Model file for the job. Use its own axes, mm. A direction names the side the tool comes from. Coordinates: 2 decimals unless noted, no trailing zeros. Write each loop counter-clockwise with the first axis right and the second up, starting at its lowest first coordinate (ties: lowest second). Pieces come first, ordered by that corner, then holes. Notation, with made-up numbers: M 84.25,35 L 128.25,35 A33 ccw 128.25,74 Z; hole C 70.5,-36.75 d7. An arc over 180 degrees is marked long. Put each result on its own line as item: value. Start each with the question number.
Q1. Cut at B-B (y = 4.75). Write the cut outline in (x, z).
Q2. Drill centre lines: line 1 along X through (y, z) = (5, -28.5); line 2 along Z through (x, y) = (-17.5, 3.75); line 3 along Y through (x, z) = (-9.5, -18.5). Where is each one in solid material? Low to high.
Q3. Drop flat-ended pins along their axis: pin 1 (1.3 mm diameter, centred on x = -3.5, y = 5, fed in from +Z); pin 2 (3 mm diameter, centred on x = -16.06, z = -31.06, fed in from -Y); pin 3 (4.5 mm diameter, centred on x = -16.06, z = -31.06, fed in from +Y). Give the stop position or say it passes through.
Q4. Pull direction Z, two halves, no side cores. Call faces 4 (the flat face through (-22.5, 5, 0)), 5 (the flat face through (0, 5, -34.026)), 6 (the cylindrical face through (23.95, 3.25, -36.5)): pulls with the +Z half, pulls with the -Z half, needs draft (parallel to the pull), parting line crosses it, or undercut.
Q5. Which spindle directions (+Z, -Z, +X, -X, +Y, -Y) get a long thin tool onto all of the face, cutting with end or side? Do faces 1 (the flat face through (0, 5, -35.026)), 2 (the cylindrical face through (-18.238, 3.254, -29.382)), 3 (the cylindrical face through (24.14, 0.9, -0.48)). Say none if no direction does.
Q6. Cut at D-D (y = 1.5). Give the number of separate pieces and of enclosed holes in the cut face, then the cut area to 3 significant figures.
Autodesk Inventor part; units mm, degrees
ref_plane "YZ Plane" through (0, 0, 0) normal (1, 0, 0) x (0, 1, 0)
ref_plane "XZ Plane" through (0, 0, 0) normal (0, 1, 0) x (-1, 0, 0)
ref_plane "XY Plane" through (0, 0, 0) normal (0, 0, 1) x (1, 0, 0)
sketch "Sketch1" plane through (0, 0, 0) normal (0, 1, 0) x (-1, 0, 0)
  line L0 (-25, 37.5) -> (25, 37.5)
  line L1 (25, 37.5) -> (25, -37.5)
  line L2 (25, -37.5) -> (-25, -37.5)
  line L3 (-25, -37.5) -> (-25, 37.5)
  line L4 (25, 37.5) -> (-25, -37.5) construction
  line L5 (-22.5, 35) -> (22.5, 35)
  line L6 (22.5, 35) -> (22.5, -35)
  line L7 (22.5, -35) -> (-22.5, -35)
  line L8 (-22.5, -35) -> (-22.5, 35)
  line L9 (22.5, 35) -> (-22.5, -35) construction
  line L10 (22.5, 35) -> (20, 35)
  line L11 (20, 35) -> (20, 32.5)
  line L12 (20, 32.5) -> (22.5, 32.5)
  line L13 (22.5, 32.5) -> (22.5, 35)
  arc A0 (22.5, 32.5) -> (20, 35) centre (20, 32.5) ccw
  line L14 (25, 37.5) -> (21.5, 37.5)
  line L15 (21.5, 37.5) -> (21.5, 34)
  line L16 (21.5, 34) -> (25, 34)
  line L17 (25, 34) -> (25, 37.5)
  line L18 (22.5, -35) -> (20, -35)
  line L19 (20, -35) -> (20, -32.5)
  line L20 (20, -32.5) -> (22.5, -32.5)
  line L21 (22.5, -32.5) -> (22.5, -35)
  line L22 (-22.5, -35) -> (-20, -35)
  line L23 (-20, -35) -> (-20, -32.5)
  line L24 (-20, -32.5) -> (-22.5, -32.5)
  line L25 (-22.5, -32.5) -> (-22.5, -35)
  line L26 (-22.5, 35) -> (-20, 35)
  line L27 (-20, 35) -> (-20, 32.5)
  line L28 (-20, 32.5) -> (-22.5, 32.5)
  line L29 (-22.5, 32.5) -> (-22.5, 35)
  arc A1 (-20, 35) -> (-22.5, 32.5) centre (-20, 32.5) ccw
  arc A2 (-22.5, -32.5) -> (-20, -35) centre (-20, -32.5) ccw
  arc A3 (20, -35) -> (22.5, -32.5) centre (20, -32.5) ccw
  arc A4 (25, 34) -> (21.5, 37.5) centre (21.5, 34) ccw
  line L30 (25, -37.5) -> (21.5, -37.5)
  line L31 (21.5, -37.5) -> (21.5, -34)
  line L32 (21.5, -34) -> (25, -34)
  line L33 (25, -34) -> (25, -37.5)
  line L34 (-25, -37.5) -> (-21.5, -37.5)
  line L35 (-21.5, -37.5) -> (-21.5, -34)
  line L36 (-21.5, -34) -> (-25, -34)
  line L37 (-25, -34) -> (-25, -37.5)
  line L38 (-25, 37.5) -> (-21.5, 37.5)
  line L39 (-21.5, 37.5) -> (-21.5, 34)
  line L40 (-21.5, 34) -> (-25, 34)
  line L41 (-25, 34) -> (-25, 37.5)
  arc A5 (-21.5, 37.5) -> (-25, 34) centre (-21.5, 34) ccw
  arc A6 (-25, -34) -> (-21.5, -37.5) centre (-21.5, -34) ccw
  arc A7 (21.5, -37.5) -> (25, -34) centre (21.5, -34) ccw
  point P0 (0, 0)
  point P1 (25, 34)
  point P2 (-25, -34)
  point P3 (-22.5, -32.5)
  point P4 (-22, -34)
  point P5 (-22.5, -34)
  point P6 (22.5, -32.5)
  dimension "d0" = 50
  dimension "d1" = 75
  dimension "d2" = 45
  dimension "d3" = 70
  dimension "d8" = 2.5
  dimension "d9" = 2.5
extrude "Extrusion3" add sketch "Sketch1" along normal blind 3.5 contours L0 L15 L5 L39 | L39 L5 L8 L40 A5 | L40 L8 L36 L3 | A4 L16 L6 L5 L15 | L39 A1 L40 L8 L5 | L5 A1 L39 | L36 L8 L7 L35 A6 | L40 A1 L8 | L15 A0 L5 | L5 L6 L16 A0 L15 | L1 L32 L6 L16 | L5 L11 L12 L6 L20 L19 L7 L23 L24 L8 L28 L27 | L27 L28 A1 L40 L39 | L39 L40 A1 | L36 A2 L35 L7 L8 | L8 A2 L36 | L35 L7 L31 L2 | A0 L15 L16 L12 L11 | A0 L16 L15 | A7 L31 L7 L6 L32 | L6 A0 L16 | L24 L23 A2 L35 L36 | L36 L35 A2 | L35 A2 L7 | L32 A3 L6 | L6 L7 L31 A3 L32 | L7 A3 L31 | A3 L32 L31 L19 L20 | A3 L31 L32
fillet "Fillet1" radius 3 8 edges at (-23.9749, 0, 36.4749) (0, 0, 37.5) (23.9749, 0, 36.4749) (25, 0, 0) (23.9749, 0, -36.4749) (0, 0, -37.5) (-23.9749, 0, -36.4749) (-25, 0, 0)
sketch "Sketch2" plane through (0, 3.5, 0) normal (0, 1, 0) x (1, 0, 0)
  arc A0 (20, 32.5) -> (17.5, 35) centre (17.5, 32.5) ccw
  line L0 (17.5, 35) -> (17.5, 33.5)
  line L1 (20, -32.5) -> (20, 32.5)
  line L2 (20, 32.5) -> (18.5, 32.5)
  line L3 (18.5, 32.5) -> (17.5, 33.5)
  line L4 (18, 33) -> (16.0555, 31.0555)
  circle A1 centre (16.0555, 31.0555) radius 2.75
  line L5 (-20, 32.5) -> (-20, -32.5)
  line L6 (-20, -32.5) -> (-18.5, -32.5)
  line L7 (-17.5, -35) -> (17.5, -35)
  line L8 (-17.5, -35) -> (-17.5, -33.5)
  line L9 (-17.5, -33.5) -> (-18.5, -32.5)
  line L10 (-18, -33) -> (-16.0555, -31.0555)
  line L11 (-18, -33) -> (-15.25, -33) construction
  circle A2 centre (-16.0555, -31.0555) radius 2.75
  arc A3 (17.5812, 28.7675) -> (18.8055, 31.0555) centre (16.0555, 31.0555) ccw construction
  arc A4 (17.8504, 28.3639) -> (19.2906, 31.0555) centre (16.0555, 31.0555) ccw
  arc A5 (17.3121, 29.1712) -> (18.3203, 31.0555) centre (16.0555, 31.0555) ccw
  arc A6 (17.3121, 29.1712) -> (17.8504, 28.3639) centre (17.5812, 28.7675) ccw
  arc A7 (19.2906, 31.0555) -> (18.3203, 31.0555) centre (18.8055, 31.0555) ccw
  arc A8 (14.2605, 33.747) -> (12.8203, 31.0555) centre (16.0555, 31.0555) ccw
  arc A9 (12.8203, 31.0555) -> (13.7906, 31.0555) centre (13.3055, 31.0555) ccw
  arc A10 (14.7989, 32.9398) -> (14.2605, 33.747) centre (14.5297, 33.3434) ccw
  arc A11 (14.7989, 32.9398) -> (13.7906, 31.0555) centre (16.0555, 31.0555) ccw
  arc A12 (-14.2605, -33.747) -> (-12.8203, -31.0555) centre (-16.0555, -31.0555) ccw
  arc A13 (-14.7989, -32.9398) -> (-13.7906, -31.0555) centre (-16.0555, -31.0555) ccw
  arc A14 (-14.7989, -32.9398) -> (-14.2605, -33.747) centre (-14.5297, -33.3434) ccw
  arc A15 (-12.8203, -31.0555) -> (-13.7906, -31.0555) centre (-13.3055, -31.0555) ccw
  arc A16 (-17.8504, -28.3639) -> (-19.2906, -31.0555) centre (-16.0555, -31.0555) ccw
  arc A17 (-19.2906, -31.0555) -> (-18.3203, -31.0555) centre (-18.8055, -31.0555) ccw
  arc A18 (-17.3121, -29.1712) -> (-17.8504, -28.3639) centre (-17.5812, -28.7675) ccw
  arc A19 (-17.3121, -29.1712) -> (-18.3203, -31.0555) centre (-16.0555, -31.0555) ccw
  line L12 (-19.2843, -34.2843) -> (-16.7157, -31.7157) construction
  line L13 (-18.86, -34.7085) -> (-16.2915, -32.14)
  line L14 (-17.14, -31.2915) -> (-19.7085, -33.86)
  arc A20 (-19.7085, -33.86) -> (-18.86, -34.7085) centre (-19.2843, -34.2843) ccw
  arc A21 (-16.2915, -32.14) -> (-17.14, -31.2915) centre (-16.7157, -31.7157) ccw
  line L15 (16.5205, 31.5205) -> (19.4795, 34.4795) construction
  line L16 (16.9448, 31.0962) -> (19.9038, 34.0552)
  line L17 (19.0552, 34.9038) -> (16.0962, 31.9448)
  arc A22 (16.0962, 31.9448) -> (16.9448, 31.0962) centre (16.5205, 31.5205) ccw
  arc A23 (19.9038, 34.0552) -> (19.0552, 34.9038) centre (19.4795, 34.4795) ccw
  circle A24 centre (16.0555, 31.0555) radius 1.25
  circle A25 centre (-16.0555, -31.0555) radius 1.25
  line L18 (21.5, 34.5) -> (-21.5, 34.5)
  line L19 (0, 34.5) -> (0, -35)
  circle A26 centre (16.0555, -31.0555) radius 2.75
  circle A27 centre (16.0555, -31.0555) radius 1.25
  circle A28 centre (-16.0555, 31.0555) radius 2.75
  circle A29 centre (-16.0555, 31.0555) radius 1.25
  point P0 (0, 0)
  point P1 (18.3774, 32.5289)
  point P2 (17.5289, 33.3774)
  point P3 (14.9555, 33.5759)
  point P4 (13.3482, 30.5722)
  point P5 (17.1554, 28.535)
  point P6 (18.7627, 31.5387)
  point P7 (-18.3774, -32.5289)
  point P8 (-17.5289, -33.3774)
  point P9 (-14.9555, -33.5759)
  point P10 (-13.3482, -30.5722)
  point P11 (-17.1554, -28.535)
  point P12 (-18.7627, -31.5387)
  dimension "d32" = 5.5
  dimension "d29" = 1.5
  dimension "d30" = 1.5
  dimension "d31" = 2.75
  dimension "d33" = 1.5
  dimension "d34" = 1.5
  dimension "d35" = 2.75
  dimension "d36" = 45
  dimension "d37" = 5.5
  dimension "d40" = 360
  dimension "d44" = 1.2
  dimension "d45" = 1.2
  dimension "d60" = 2.5
  dimension "d61" = 2.5
sketch "Sketch4" plane through (0, 3.5, 0) normal (0, 1, 0) x (1, 0, 0)
  line L0 (-22, 34.5263) -> (22, 34.5263)
  line L1 (22, 34.5263) -> (22, -34.5263)
  line L2 (22, -34.5263) -> (-22, -34.5263)
  line L3 (-22, -34.5263) -> (-22, 34.5263)
  line L4 (-22, 34.5263) -> (22, -34.5263) construction
  line L5 (22, 34.5263) -> (-22, -34.5263) construction
  line L6 (21.5, 34.5) -> (-21.5, 34.5)
  line L7 (-21.5, 34.5) -> (-21.5, 37.5)
  line L8 (17.5001, 34.5) -> (-21.5, 34.5) construction
  line L9 (22, -34) -> (22, 34)
  line L10 (22, 32.5003) -> (22, -34.5263) construction
  arc A0 (21.5, -34.5263) -> (22.5, -34.5263) centre (22, -34.5263) ccw
  line L11 (22, -34.5263) -> (-22, -34.5263) construction
  line L12 (22, -34.0263) -> (-22, -34.0263)
  line L13 (-22, -35.0263) -> (22, -35.0263)
  arc A1 (22, -35.0263) -> (22, -34.0263) centre (22, -34.5263) ccw
  arc A2 (-22, -34.0263) -> (-22, -35.0263) centre (-22, -34.5263) ccw
  line L14 (-22, -34.5263) -> (-22, 34.5263) construction
  line L15 (-21.5, -34.5263) -> (-21.5, 34.5263)
  line L16 (-22.5, 34.5263) -> (-22.5, -34.5263)
  arc A3 (-22.5, -34.5263) -> (-21.5, -34.5263) centre (-22, -34.5263) ccw
  arc A4 (-21.5, 34.5263) -> (-22.5, 34.5263) centre (-22, 34.5263) ccw
  line L17 (22, 34.5263) -> (-22, 34.5263) construction
  line L18 (22, 35.0263) -> (-22, 35.0263)
  line L19 (-22, 34.0263) -> (22, 34.0263)
  arc A5 (22, 34.0263) -> (22, 35.0263) centre (22, 34.5263) ccw
  arc A6 (-22, 35.0263) -> (-22, 34.0263) centre (-22, 34.5263) ccw
  line L20 (22, -34.5263) -> (22, 34.5263) construction
  line L21 (22.5, -34.5263) -> (22.5, 34.5263)
  line L22 (21.5, 34.5263) -> (21.5, -34.5263)
  arc A7 (21.5, -34.5263) -> (22.5, -34.5263) centre (22, -34.5263) ccw
  arc A8 (22.5, 34.5263) -> (21.5, 34.5263) centre (22, 34.5263) ccw
  point P0 (0, 0)
  point P1 (-1.9999, 34.5)
  point P2 (22, -1.013)
  point P3 (0, -34.5263)
  point P4 (-22, 0)
  point P5 (0, 34.5263)
  point P6 (22, 0)
  point P7 (-22.5, -34.5263)
  point P8 (22, -35.0263)
  point P9 (22.5, -34.5263)
  point P10 (22.5, 34.5263)
  point P11 (-21.5, -34.0263)
  point P12 (-21.5, 34.0263)
  point P13 (21.5, 34.0263)
  point P14 (21.5, -34.0263)
  dimension "d68" = 1
  dimension "d69" = 1
  dimension "d70" = 1
  dimension "d71" = 1
  dimension "d72" = 1
extrude "Extrusion11" add sketch "Sketch4" along normal blind 3 contours L3 A6 A4 L0 | L0 L7 L15 L19 L3 | L7 L18 A8 L0 | L0 L22 L6 L7 | A4 L18 L7 | L19 L15 L12 L3 | L3 A2 L16 A6 | A8 A5 L1 L0 | L0 L1 L19 L22 | L6 L22 L19 L15 | L12 L15 L2 L3 | L3 L2 A3 A2 | L12 L22 L2 L15 | L19 L1 L12 L22 | A5 L21 A1 L1 | L2 A0 L13 A3 | L12 L1 L2 L22 | A0 L2 L1 A1
fillet "Fillet2" radius 0.5 12 edges at (-22.3536, 6.5, -34.8799) (-22.5, 6.5, 0) (-22.3536, 6.5, 34.8799) (0, 6.5, 35.0263) (22.3536, 6.5, 34.8799) (22.5, 6.5, 0) (22.3536, 6.5, -34.8799) (0, 6.5, -35.0263) (0, 6.5, -34.0263) (21.5, 6.5, 0) (0, 6.5, 34.0263) (-21.5, 6.5, 0)
extrude "Extrusion12" cut sketch "Sketch2" against normal blind 0.5 contours A26 | A28
sketch "Sketch6" plane through (0, 3.5, 0) normal (0, 1, 0) x (1, 0, 0)
  circle A0 centre (16.0555, -31.0555) radius 1.25
  circle A1 centre (16.0555, -31.0555) radius 1.25
  point P0 (0, 0)
extrude "Extrusion13" cut sketch "Sketch6" against normal blind 5
sketch "Sketch7" plane through (-16.0555, 3.5, -31.0555) normal (0, 1, 0) x (1, 0, 0)
  circle A0 centre (0, 0) radius 1.25
  point P0 (16.0555, -31.0555)
extrude "Extrusion14" cut sketch "Sketch7" against normal blind 5
chamfer "Chamfer2" distance 0.5 angle 45 2 edges at (14.8055, 0, 31.0555) (-17.3055, 0, -31.0555)
properties part number "proper shit spodnji"
Computed values:
1. outline: M -22.5,-34.53 A0.5 ccw -22,-35.03 L 22,-35.03 A0.5 ccw 22.5,-34.53 L 22.5,34.53 A0.5 ccw 22,35.03 L -22,35.03 A0.5 ccw -22.5,34.53 Z; hole M -21.5,-34.03 L 21.5,-34.03 L 21.5,34.03 L -21.5,34.03 Z
2. line 1: -22.5 to -21.5, 21.5 to 22.5
2. line 2: -35.03 to -34.03, 34.03 to 35.03
2. line 3: 0 to 3.5
3. pin 1: z = 35.03
3. pin 2: y = 0.24
3. pin 3: y = 3
4. face 4: needs draft
4. face 5: undercut
4. face 6: pulls with the -Z half
5. face 1: -Z, +X, -X, +Y
5. face 2: +Y
5. face 3: +Z, -Z, +X, -Y
6. separate pieces: 1
6. enclosed holes: 2
6. area: 3,630 mm2
